The listing builds one solid part. Answer for the finished solid, in the listing's coordinates (mm). A direction names the side the tool comes from. Round coordinates to 2 decimals unless told otherwise and drop trailing zeros. Order: outer loops, then holes, each group sorted by start corner. A loop starts at its lowest first (then second) coordinate and runs counter-clockwise, first axis right, second up. Notation, with made-up numbers: (-39, 77.25) -> (-4, 77.25) arc R29 ccw to (-4, 111.25) -> close; hole circle Ø6 at (-4, 26.25). An arc over 180 degrees is marked (long way). Return JSON: item names as keys, results as strings. Group by question number.
(1) Each of these flat-tipped pins is pushed along its axis until it touches: pin 1 (0.6 mm diameter, centred on x = -4.5, y = -2.5, fed in from +Z); pin 2 (5 mm diameter, centred on x = 1, y = -0.5, fed in from -Z); pin 3 (2 mm diameter, centred on x = 2.5, z = 1.5, fed in from +Y) (3 decimals); pin 4 (2 mm diameter, centred on x = 0, y = 0, fed in from -Z). Where does it stop, or does it pass through?
(2) The part is cut by section B-B (x = 0). Determine the outline of the cut face in (y, z), plus the area to 3 significant figures.
(3) Consider line 1 (X direction, y = 0, z = 1.5); line 2 (Y direction, x = 0, z = 1.9); line 3 (Z direction, x = -2, y = -0.5). Determine where each line is inside the solid, lowest interval first. Write a range as [from, to].
(4) The part is cut by section C-C (y = -4.5). Determine the outline of the cut face in (x, z) (1 decimal).
(5) Which of the six approach directions +Z, -Z, +X, -X, +Y, -Y give full straight-line access (tool end or side, diameter ignored) to faces 1 (the face through (5.1, 4.8, 0.5)), 2 (the face through (3.9, 5, 2)), 3 (the face through (-3.9, -5, 2)), 4 (the face through (-0.83, 5.174, 0.129)), 5 (the face through (0.48, 2.86, -0.52))?
(6) Determine the mould class of faces 6 (the face through (-5.1, -5, 0.5)), 7 (the face through (-2, 0, 2.2)), 8 (the face through (1.4, -1.3, 1)) for opening direction X: +X half, -X half, draft (parallel to the pull), parting line (faces both ways), or undercut.
(7) The part is cut by section A-A (z = 0.65). Determine the outline of the cut face in (x, y), plus the area to 3 significant figures.
(8) The part is cut by section D-D (x = 2.5). Determine the outline of the cut face in (y, z), plus the area to 3 significant figures.
from build123d import *

# Parameters (mm, degrees)
PAD_DEPTH       = 12.5
POCKET_DEPTH    = 4.201
SKETCH003_R     = 1.75
POCKET001_DEPTH = 4.201
POCKET002_DEPTH = 3
FILLET_R        = 1


with BuildPart() as part:
    # Sketch → Pad (new body, symmetric)
    with BuildSketch(Plane.XZ):
        with BuildLine():
            Line((-3.9, 2.2), (3.9, 2.2))
            Line((3.9, 2.2), (3.9, 1))
            Line((3.9, 1), (5.1, 1))
            Line((5.1, 1), (5.1, 0))
            ThreePointArc((-5.1, 0), (0, -2), (5.1, 0))
            Line((-5.1, 0), (-5.1, 1))
            Line((-5.1, 1), (-3.9, 1))
            Line((-3.9, 1), (-3.9, 2.2))
        make_face()
    extrude(amount=PAD_DEPTH, both=True)

    # Sketch002 (on Face4 of Pad) → Pocket (cut, through all)
    with BuildSketch(Plane(origin=(0, 0, 2.2), x_dir=(-1, 0, 0), z_dir=(0, 0, 1))):
        Polygon((-5.1, -0.102052), (5.1, 12.5), (-5.1, 12.5), align=None)
        Polygon((-5.1, -12.5), (5.1, 0.102052), (5.1, -12.5), align=None)
    extrude(amount=-POCKET_DEPTH, mode=Mode.SUBTRACT)

    # Sketch003 (on Face8 of Pocket) → Pocket001 (cut, through all)
    with BuildSketch(Plane(origin=(0, 0, 2.2), x_dir=(-1, 0, 0), z_dir=(0, 0, 1))):
        Circle(SKETCH003_R)
    extrude(amount=-POCKET001_DEPTH, mode=Mode.SUBTRACT)

    # Sketch004 (on DatumPlane) → Pocket002 (cut)
    with BuildSketch(Plane.XY.offset(-2)):
        Polygon((3.308847, -0.523478), (2.107769, 2.603807), (-1.201078, 3.127285), (-3.308847, 0.523478), (-2.107769, -2.603807), (1.201078, -3.127285), align=None)
    extrude(amount=POCKET002_DEPTH, mode=Mode.SUBTRACT)

    # Fillet
    fillet_edges = [part.edges().sort_by_distance(p)[0] for p in [
        (5.1, 12.5, 0.5),
        (-5.1, -12.5, 0.5),
    ]]
    fillet(fillet_edges, radius=FILLET_R)


solid = part.part
Answer below:
{
 "1": {"pin 1": "stops at z = 1", "pin 2": "stops at z = -1.88", "pin 3": "stops at y = 10.475", "pin 4": "passes through"},
 "2": {"outline": "(-6.2, -2) -> (-2.94, -2) -> (-2.94, 1) -> (-1.75, 1) -> (-1.75, 2.2) -> (-6.2, 2.2) -> close; (1.75, 1) -> (2.94, 1) -> (2.94, -2) -> (6.2, -2) -> (6.2, 2.2) -> (1.75, 2.2) -> close", "area": "30.2 mm²"},
 "3": {"line 1": "x = [-3.9, -1.75], [1.75, 3.9]", "line 2": "y = [-6.2, -1.75], [1.75, 6.2]", "line 3": "z = [1, 2.2]"},
 "4": {"outline": "(-5.1, 0) arc R7.5 ccw to (1.4, -1.9) -> (1.4, 2.2) -> (-3.9, 2.2) -> (-3.9, 1) -> (-5.1, 1) -> close"},
 "5": {"face 1": "+Z, -Z, +X, +Y, -Y", "face 2": "+Z, +X, +Y, -Y", "face 3": "+Z, -X, +Y, -Y", "face 4": "+Z, -Z, -X, +Y", "face 5": "-Z"},
 "6": {"face 6": "-X half", "face 7": "draft", "face 8": "undercut"},
 "7": {"outline": "(-5.1, -9.68) arc R1 ccw to (-3.32, -10.3) -> (5.1, 0.1) -> (5.1, 9.68) arc R1 ccw to (3.32, 10.3) -> (-5.1, -0.1) -> close; hole (-3.31, 0.52) -> (-2.11, -2.6) -> (1.2, -3.13) -> (3.31, -0.52) -> (2.11, 2.6) -> (-1.2, 3.13) -> close", "area": "94.1 mm²"},
 "8": {"outline": "(-3.11, -1.57) -> (-1.52, -1.57) -> (-1.52, 1) -> (1.58, 1) -> (1.58, -1.57) -> (9.29, -1.57) -> (9.29, 2.2) -> (-3.11, 2.2) -> close", "area": "38.8 mm²"}
}
